Work out the finished part from the listing and answer in its coordinate system (mm). A direction names the side the tool comes from. Round coordinates to 2 decimals unless told otherwise and drop trailing zeros. Order: outer loops, then holes, each group sorted by start corner. A loop starts at its lowest first (then second) coordinate and runs counter-clockwise, first axis right, second up. Notation, with made-up numbers: (-13, 33) - (31, 33) arc R12 cw to (31, 50) - close; hole circle Ø9 at (5.5, -33.75). An arc over 180 degrees is marked (long way). Use CSV: the item, a comma, the result in double quotes.
from build123d import *

# Parameters (mm, degrees)
ESQUISSE1_W        = 50
ESQUISSE1_H        = 83
ESQUISSE1_R        = 1.5
BOSS_EXTRU_1_DEPTH = 1.6
ESQUISSE2_R        = 6.5
BOSS_EXTRU_2_DEPTH = 20.5


with BuildPart() as part:
    # Esquisse1 → Boss.-Extru.1 (new body)
    with BuildSketch(Plane.XY):
        with Locations((25, -41.5)):
            Rectangle(ESQUISSE1_W, ESQUISSE1_H)
        with Locations((3, -3)):
            Circle(ESQUISSE1_R, mode=Mode.SUBTRACT)
        with Locations((47, -3)):
            Circle(ESQUISSE1_R, mode=Mode.SUBTRACT)
        with Locations((47, -80)):
            Circle(ESQUISSE1_R, mode=Mode.SUBTRACT)
        with Locations((3, -80)):
            Circle(ESQUISSE1_R, mode=Mode.SUBTRACT)
    extrude(amount=BOSS_EXTRU_1_DEPTH)

    # Esquisse2 → Boss.-Extru.2 (add)
    with BuildSketch(Plane.XY.offset(1.6)):
        with Locations((7, -29)):
            Circle(ESQUISSE2_R)
        with Locations((43, -29)):
            Circle(ESQUISSE2_R)
    extrude(amount=BOSS_EXTRU_2_DEPTH)


solid = part.part
(1) Find the intervals of material crossed by L1, parallel to X at y = -80, z = 0.4; L2, parallel to Y at x = 47, z = 0.95; L3, parallel to Z at x = 28, y = -34.5, in increasing order. Write a range as from..to.
Findings below:
L1,"x = 0..1.5, 4.5..45.5, 48.5..50"
L2,"y = -83..-81.5, -78.5..-4.5, -1.5..0"
L3,"z = 0..1.6"
(2) Find section C-C (z = 6.5). Determine the outline of the cut face in (x, y), and give its area (3 significant figures).
Findings below:
outline,"circle Ø13 at (7, -29); circle Ø13 at (43, -29)"
area,"265 mm²"
(3) For faces 1 (the cylindrical face through (36.506, -28.714, 11.706)), 2 (the cylindrical face through (3.806, -78.735, 0.789)), determine the directions among +Z, -Z, +X, -X, +Y, -Y from which every point of the face is accessible in a straight line to the end or side of a thin tool.
Findings below:
face 1,"+Z"
face 2,"+Z, -Z"
(4) The mould has two halves that part along Y. Classify faces 3 (the flat face through (43, -29, 22.1)), 4 (the cylindrical face through (10.494, -23.519, 11.706)), 5 (the cylindrical face through (3.806, -1.735, 0.789)): released by +Y, released by -Y, zero draft, split by the parting line, or undercut.
Findings below:
face 3,"zero draft"
face 4,"split by the parting line"
face 5,"undercut"
(5) Each of these flat-tipped pins is pushed along its axis until it touches: pin 1 (10 mm diameter, centred on x = 10.5, z = 17.5, fed in from +Y); pin 2 (1.5 mm diameter, centred on y = -49, z = 2.5, fed in from -X); pin 3 (5 mm diameter, centred on x = 34.5, z = 12.5, fed in from -Y); pin 4 (3.5 mm diameter, centred on x = 47, y = -3, fed in from -Z). Where does it stop, or does it pass through?
Findings below:
pin 1,"stops at y = -22.5"
pin 2,"passes through"
pin 3,"stops at y = -31.5"
pin 4,"stops at z = 0"
(6) Find section D-D (y = -29). Determine the outline of the cut face in (x, z), and give its area (3 significant figures).
Findings below:
outline,"(0, 0) - (50, 0) - (50, 1.6) - (49.5, 1.6) - (49.5, 22.1) - (36.5, 22.1) - (36.5, 1.6) - (13.5, 1.6) - (13.5, 22.1) - (0.5, 22.1) - (0.5, 1.6) - (0, 1.6) - close"
area,"613 mm²"
(7) Find section A-A (y = -80). Determine the outline of the cut face in (x, z), and give its area (3 significant figures).
Findings below:
outline,"(0, 0) - (1.5, 0) - (1.5, 1.6) - (0, 1.6) - close; (4.5, 0) - (45.5, 0) - (45.5, 1.6) - (4.5, 1.6) - close; (48.5, 0) - (50, 0) - (50, 1.6) - (48.5, 1.6) - close"
area,"70.4 mm²"
(8) Find section B-B (x = 47). Determine the outline of the cut face in (y, z), and give its area (3 significant figures).
Findings below:
outline,"(-83, 0) - (-81.5, 0) - (-81.5, 1.6) - (-83, 1.6) - close; (-78.5, 0) - (-4.5, 0) - (-4.5, 1.6) - (-23.88, 1.6) - (-23.88, 22.1) - (-34.12, 22.1) - (-34.12, 1.6) - (-78.5, 1.6) - close; (-1.5, 0) - (0, 0) - (0, 1.6) - (-1.5, 1.6) - close"
area,"333 mm²"
